Model file for the job. Use its own axes, mm. Face numbers are marked on the shaded views. A direction names the side the tool comes from. Round coordinates to 2 decimals unless told otherwise and drop trailing zeros. Write each loop counter-clockwise with the first axis right and the second up, starting at its lowest first coordinate (ties: lowest second). Pieces come first, ordered by that corner, then holes. Notation, with made-up numbers: (15.25, 18) - (67.25, 18) arc R24 ccw to (67.25, 53) - close; hole circle Ø10 at (-1.5, 55). An arc over 180 degrees is marked (long way). Answer as a JSON object with one key per item and string values. Group by question number.
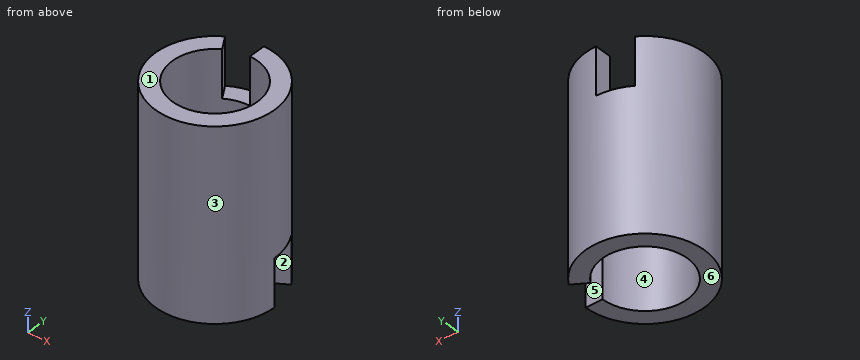
from build123d import *

# Parameters (mm, degrees)
BOSS_EXTRUDE1_DEPTH      = 10
BOSS_EXTRUDE1_DEPTH_BACK = 10
SKETCH1_R                = 6.5
SKETCH1_R_2              = 4.5
CUT_EXTRUDE2_DEPTH       = 5
SKETCH4_R                = 6.5
SKETCH4_R_2              = 6.3
CUT_EXTRUDE4_DEPTH       = 23.011360703
CUT_EXTRUDE3_DEPTH       = 5


with BuildPart() as part:
    # Sketch1 → Boss-Extrude1 (new, two sides: drawn at the far end of the back side and taken through both)
    with BuildSketch(Plane.XY.offset(-BOSS_EXTRUDE1_DEPTH_BACK)):
        Circle(SKETCH1_R)
        Circle(SKETCH1_R_2, mode=Mode.SUBTRACT)
    extrude(amount=BOSS_EXTRUDE1_DEPTH + BOSS_EXTRUDE1_DEPTH_BACK)

    # Sketch2 → Cut-Extrude2 (cut)
    with BuildSketch(Plane.XY.offset(10)):
        with BuildLine():
            Line((-6.230040483, 9.970148902), (0, 0))
            Line((0, 0), (0, 11.756584264))
            ThreePointArc((0, 11.756584264), (-3.2405538, 11.301154128), (-6.230040483, 9.970148902))
        make_face()
    extrude(amount=-CUT_EXTRUDE2_DEPTH, mode=Mode.SUBTRACT)

    # Sketch4 → Cut-Extrude4 (cut, through all)
    with BuildSketch(Plane.XY.offset(10)):
        Circle(SKETCH4_R)
        Circle(SKETCH4_R_2, mode=Mode.SUBTRACT)
    extrude(amount=-CUT_EXTRUDE4_DEPTH, mode=Mode.SUBTRACT)

    # Sketch3 → Cut-Extrude3 (cut)
    with BuildSketch(Plane.XY.offset(-10)):
        with BuildLine():
            Line((9.970148902, 6.230040483), (0, 0))
            Line((0, 0), (11.756584264, 0))
            ThreePointArc((11.756584264, 0), (11.301154128, 3.2405538), (9.970148902, 6.230040483))
        make_face()
    extrude(amount=CUT_EXTRUDE3_DEPTH, mode=Mode.SUBTRACT)


solid = part.part
(1) Pull direction X, two halves, no side cores. Call the marked faces 1, 2, 3 and 4: pulls with the +X half, pulls with the -X half, needs draft (parallel to the pull), parting line crosses it, or undercut.
(2) Slice it at B-B (x = 4.25). Write the cut outline in (y, z), then the cut area to 3 significant figures.
(3) Slice it at C-C (z = 5.25). Write the cut outline in (x, y), then the cut area to 3 significant figures.
(4) Drill centre lines: line 1 (X direction, y = 0, z = 1); line 2 (X direction, y = -1.25, z = 7.25). Where is each one in solid material? Low to high. Write a range as from..to.
(5) 3-axis set-ups, long thin cutter, end or side, ignore diameter. For the marked faces 5 and 6: which of +Z, -Z, +X, -X, +Y, -Y reach the whole face in a straight line?
(6) Flat gauge pins, fed straight in: pin 1 (1.4 mm diameter, centred on x = 5, z = -8.5, fed in from +Y); pin 2 (5 mm diameter, centred on y = -4.5, z = 4.5, fed in from -X); pin 3 (0.7 mm diameter, centred on x = -1, y = 5.5, fed in from +Z); pin 4 (2.5 mm diameter, centred on x = 4.5, y = 2, fed in from -Z). Where does each tip first touch, or does it go through?
(7) Slice it at A-A (y = 0.25). Write the cut outline in (x, z), then the cut area to 3 significant figures.
(8) Slice it at D-D (z = 1.5). Write the cut outline in (x, y), then the cut area to 3 significant figures.
Answer:
{
 "1": {"face 1": "needs draft", "face 2": "pulls with the +X half", "face 3": "parting line crosses it", "face 4": "undercut"},
 "2": {"outline": "(-4.65, -10) - (-1.48, -10) - (-1.48, 10) - (-4.65, 10) - close; (1.48, -5) - (2.66, -5) - (2.66, -10) - (4.65, -10) - (4.65, 10) - (1.48, 10) - close", "area": "121 mm²"},
 "3": {"outline": "(-3.34, 5.34) arc R6.3 ccw (long way) to (0, 6.3) - (0, 4.5) arc R4.5 cw (long way) to (-2.38, 3.82) - close", "area": "55.6 mm²"},
 "4": {"line 1": "-6.3..-4.5, 4.5..6.3", "line 2": "-6.17..-4.32, 4.32..6.17"},
 "5": {"face 5": "-Z, +X", "face 6": "-Z, +X, -X, +Y, -Y"},
 "6": {"pin 1": "y = 4.6", "pin 2": "x = -5.97", "pin 3": "z = 5", "pin 4": "z = -10"},
 "7": {"outline": "(-6.3, -10) - (-4.49, -10) - (-4.49, 10) - (-6.3, 10) - close; (4.49, -5) - (6.3, -5) - (6.3, 10) - (4.49, 10) - close", "area": "63.1 mm²"},
 "8": {"outline": "circle Ø12.6 at (0, 0); hole circle Ø9 at (0, 0)", "area": "61.1 mm²"}
}
